```python
from build123d import *

# Parameters (mm, degrees)
SKETCH1_W             = 43.18
SKETCH1_H             = 48.26
BASE_DEPTH            = 4.7625
MOTORHOLES_AT_2_COUNT = 2
MOTORHOLES_AT_2_PITCH = 11.43
MOTORHOLES_AT_3_COUNT = 2
MOTORHOLES_AT_3_PITCH = 43.30603911
MOTORHOLES_AT_4_COUNT = 2
MOTORHOLES_AT_4_PITCH = 39.703669394


with BuildPart() as part:
    # Sketch1 → Base (new body)
    with BuildSketch(Plane(origin=(0, 0, 0), x_dir=(1, 0, 0), z_dir=(0, 1, 0))):
        Rectangle(SKETCH1_W, SKETCH1_H)
    extrude(amount=BASE_DEPTH)

    # Sketch2 → MotorHoles (revolve, cut)
    with BuildSketch(Plane(origin=(5.715, 0, 19.5072), x_dir=(0, 0, -1), z_dir=(1, 0, 0))):
        Polygon((0, 0), (0, 4.7625), (1.63195, 4.7625), (1.63195, 1.7272), (3.37312, 1.7272), (3.37312, 0.635), (4.00812, 0), align=None)
    motorholes = revolve(axis=Axis((5.715, -6.35, 19.5072), (0, 1, 0)), mode=Mode.SUBTRACT)

    # MotorHoles at 2: MotorHoles ×2
    with Locations(*[(-i * MOTORHOLES_AT_2_PITCH, 0, 0) for i in range(1, MOTORHOLES_AT_2_COUNT)]):
        add(motorholes, mode=Mode.SUBTRACT)

    # MotorHoles at 3: MotorHoles ×2
    with Locations(*[Vector(-0.43402722545097383, 0, -0.9008997544495889) * (i * MOTORHOLES_AT_3_PITCH) for i in range(1, MOTORHOLES_AT_3_COUNT)]):
        add(motorholes, mode=Mode.SUBTRACT)

    # MotorHoles at 4: MotorHoles ×2
    with Locations(*[Vector(0.1855244140503859, 0, -0.9826396551082502) * (i * MOTORHOLES_AT_4_PITCH) for i in range(1, MOTORHOLES_AT_4_COUNT)]):
        add(motorholes, mode=Mode.SUBTRACT)


solid = part.part
```
Work out the finished part from the listing and answer in its coordinate system (mm). A direction names the side the tool comes from. Give positions to 0.01 mm unless a question says otherwise; leave off trailing zeros. Loops run counter-clockwise (first coordinate to the right, second up) from the corner with the lowest first, then second, coordinate; pieces in that order, holes last. Notation, with made-up numbers: (85.25, -16) -> (101.25, -16) arc R7 cw to (101.25, -7) -> close; hole circle Ø10 at (11.5, 51). An arc over 180 degrees is marked (long way). Put each result on its own line as item: value. Start each with the question number.
Item 1: The part is cut by section B-B (z = 19). State how many separate pieces and enclosed holes the cut face has, then the cut area to 3 significant figures.
Item 2: Each of these flat-tipped pins is pushed along its axis until it touches: P1, Ø3, axis at x = 13.08, z = -19.51, coming from the +Y side; P2, Ø5, axis at x = -5.72, z = 19.51, coming from the -Y side. Where does it stop, or does it pass through?
Item 3: Which of the six approach directions +Z, -Z, +X, -X, +Y, -Y give full straight-line access (tool end or side, diameter ignored) to faces 4 (the face through (-6.82, 3.22, 20.71)), 5 (the face through (-11.03, 1.17, -16.83))?
Item 4: The mould has two halves that part along X. Classify faces 1 (the face through (6.71, 3.22, 20.8)), 2 (the face through (0, 2, -24.13)), 3 (the face through (21.59, 2, 0)): released by +X, released by -X, zero draft, split by the parting line, or undercut.
Item 5: The part is cut by section A-A (y = 4). Give the vertices of the cut face in (x, z) (3 decimals).
Item 6: Find the intervals of material crossed by L1, parallel to X at y = 1.2, z = 22.5; L2, parallel to X at y = 0.25, z = -20; L3, parallel to Z at x = -15.5, y = 1.45, in increasing order. Write a range as [from, to].
Answers below:
1. separate pieces: 3
1. enclosed holes: 0
1. area: 163 mm2
2. P1: through
2. P2: y = 1.73
3. face 4: +Y, -Y
3. face 5: -Y
4. face 1: undercut
4. face 2: zero draft
4. face 3: released by +X
5. outline: (-21.59, -24.13) -> (21.59, -24.13) -> (21.59, 24.13) -> (-21.59, 24.13) -> close; hole circle Ø3.264 at (-13.081, -19.507); hole circle Ø3.264 at (-5.715, 19.507); hole circle Ø3.264 at (5.715, 19.507); hole circle Ø3.264 at (13.081, -19.507)
6. L1: [-21.59, -7.27], [-4.16, 4.16], [7.27, 21.59]
6. L2: [-21.59, -16.81], [-9.36, 9.36], [16.81, 21.59]
6. L3: [-24.13, -21.86], [-17.16, 24.13]
